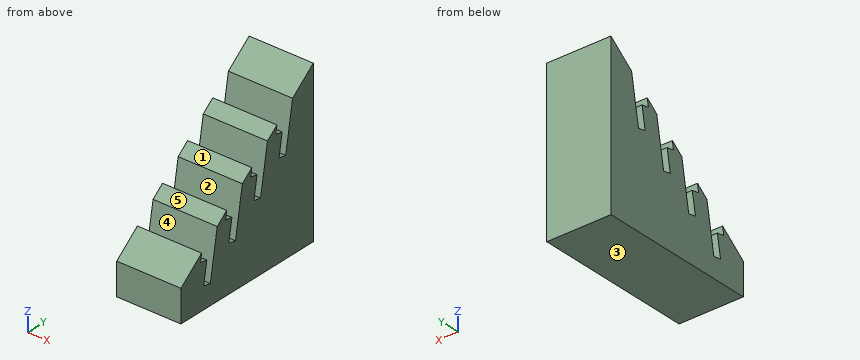
from build123d import *

# Parameters (mm, degrees)
F2_DEPTH = 25.4
F3_DEPTH = 25.4


with BuildPart() as f2:
    # F0 (on Right) → F2 (new body)
    with BuildSketch(Plane.YZ):
        Polygon((0, 12.7), (0, 0), (63.5, 0), (63.5, 63.5), align=None)
    extrude(amount=F2_DEPTH)

    # F1 (on Right) → F3 (cut)
    with BuildSketch(Plane.YZ):
        Polygon((17.4239271212, 26.6391416969), (9.9170338799, 20.6336271039), (9.3657009158, 17.5068624881), (12.4174231809, 16.9687615152), (10.91412237, 8.4431189573), (14.1159293366, 7.8785540021), align=None)
        Polygon((29.4769401208, 36.2815520967), (21.9700468796, 30.2760375036), (21.4187139155, 27.1492728878), (24.4704361805, 26.6111719149), (22.9671353697, 18.085529357), (26.1689423363, 17.5209644018), align=None)
        Polygon((41.5299531204, 45.9239624964), (34.0230598792, 39.9184479033), (33.4717269151, 36.7916832875), (36.5234491801, 36.2535823146), (35.0201483693, 27.7279397567), (38.2219553359, 27.1633748015), align=None)
        Polygon((53.5829661201, 55.5663728961), (46.0760728788, 49.5608583031), (45.5247399147, 46.4340936872), (48.5764621798, 45.8959927143), (47.0731613689, 37.3703501564), (50.2749683355, 36.8057852012), align=None)
    extrude(amount=F3_DEPTH, mode=Mode.SUBTRACT)


solid = f2.part
Can you work these out from the model? Positions are in its coordinate system, mm. Face numbers are marked on the shaded views. A direction names the side the tool comes from. Coordinates: 2 decimals unless noted, no trailing zeros. Loops run counter-clockwise (first coordinate to the right, second up) from the corner with the lowest first, then second, coordinate; pieces in that order, holes last. Notation, with made-up numbers: (-25.75, -31.5) - (27.25, -31.5) arc R25 cw to (27.25, -5.5) - close; hole circle Ø8 at (50, -23.75). An arc over 180 degrees is marked (long way). Put each result on its own line as item: value. Start each with the question number.
Item 1: If I drill on line 1 along Y through (x, z) = (24, 19) (3 decimals); line 2 along Y through (x, z) = (2, 44.5); line 3 along Y through (x, z) = (11.5, 36), over which ranges is the centre line in solid material (lowest first)?
Item 2: If we mould it in two halves opening along Y, with no side actions, what happens to the marked faces 1, 2 and 3? For each: +Y half, -Y half, draft (parallel to the pull), parting line (faces both ways), or undercut.
Item 3: Suppose I cut it at C-C (y = 19). Please give me the cut outline in (x, z).
Item 4: Suppose I cut it at A-A (z = 10.5). Please give me the cut outline in (x, y), and give its area (3 significant figures).
Item 5: Suppose I cut it at D-D (z = 23). Please give me the cut outline in (x, y).
Item 6: Suppose I cut it at B-B (x = 11.5). Please give me the cut outline in (y, z).
Item 7: Which directions (+Z, -Z, +X, -X, +Y, -Y) give clear straight access to the entire face, cutting with the end or side of a thin tool? Please do the marked faces 4 and 5.
Item 8: For pin 1 (1.5 mm diameter, centred on x = 21.5, z = 27.5, fed in from -Y); pin 2 (2 mm diameter, centred on x = 18, z = 56.5, fed in from -Y), each with a flat end and sliding along its axis, tell me the tip position at first contact or that it passes through.
Here are the results:
1. line 1: 7.875 to 9.629, 16.077 to 23.128, 26.43 to 63.5
1. line 2: 41.28 to 48.33, 51.63 to 63.5
1. line 3: 29.43 to 36.48, 39.78 to 63.5
2. face 1: -Y half
2. face 2: undercut
2. face 3: draft
3. outline: (0, 0) - (25.4, 0) - (25.4, 27.9) - (0, 27.9) - close
4. outline: (0, 0) - (25.4, 0) - (25.4, 11.28) - (0, 11.28) - close; (0, 14.58) - (25.4, 14.58) - (25.4, 63.5) - (0, 63.5) - close
4. area: 1,530 mm²
5. outline: (0, 16.78) - (25.4, 16.78) - (25.4, 23.83) - (0, 23.83) - close; (0, 27.14) - (25.4, 27.14) - (25.4, 63.5) - (0, 63.5) - close
6. outline: (0, 0) - (63.5, 0) - (63.5, 63.5) - (53.58, 55.57) - (50.27, 36.81) - (47.07, 37.37) - (48.58, 45.9) - (45.52, 46.43) - (46.08, 49.56) - (41.53, 45.92) - (38.22, 27.16) - (35.02, 27.73) - (36.52, 36.25) - (33.47, 36.79) - (34.02, 39.92) - (29.48, 36.28) - (26.17, 17.52) - (22.97, 18.09) - (24.47, 26.61) - (21.42, 27.15) - (21.97, 30.28) - (17.42, 26.64) - (14.12, 7.88) - (10.91, 8.44) - (12.42, 16.97) - (9.37, 17.51) - (9.92, 20.63) - (0, 12.7) - close
7. face 4: +Z, +X, -X
7. face 5: +Z, +X, -X, -Y
8. pin 1: y = 17.56
8. pin 2: y = 53.57
